Source: CAD feature listing. Evaluate the final solid. Frame: model axes, mm. A direction names the side the tool comes from. Round coordinates to 2 decimals unless told otherwise and drop trailing zeros. Order: outer loops, then holes, each group sorted by start corner. A loop starts at its lowest first (then second) coordinate and runs counter-clockwise, first axis right, second up. Notation, with made-up numbers: (27.5, 22) -> (62.5, 22) arc R16 ccw to (62.5, 27) -> close; hole circle Ø10 at (29.25, 61). An arc over 180 degrees is marked (long way). Write item = value, one per line. Start each with the question number.
(1) Ray query, line 1 (Z direction, x = 0, y = 1.8); line 2 (X direction, y = 2.8, z = 30); line 3 (X direction, y = 4.25, z = -30). Return the intervals inside material, ascending.
(2) Cut plane B-B on z = 0. Return the cut outline in (x, y), then the cut area to 3 significant figures.
(3) Draft query along X for faces 3 (the face through (-6.5, 6, -1)), 4 (the face through (0, 3, -40)), 5 (the face through (9.888, 6.147, -39.857)). Return one class per face: released by +X, released by -X, zero draft, split by the parting line, or undercut.
(4) Reachability of faces 1 (the face through (-9.888, 6.147, 39.857)), 2 (the face through (-3, 4, 1)) from +Z, -Z, +X, -X, +Y, -Y: full face, straight path, thin tool, end or side. Return the list, or none.
(5) Cut plane D-D on z = -22.5. Return the cut outline in (x, y).
(6) Cut plane A-A on x = 0. Give the number of separate pieces and of enclosed holes in the cut face, then the cut area to 3 significant figures.
(7) Contact query for flat-ended pins moving along their axis: pin 1 Ø4 at (x, z) = (1, 6) entering from +Y; pin 2 Ø2 at (y, z) = (5.5, -12) entering from -X; pin 3 Ø4.5 at (x, z) = (0, -30) entering from +Y. Output: stop coordinate, or through.
(8) Cut plane C-C on y = 2.5. Return the cut outline in (x, z), then the cut area to 3 significant figures.
from build123d import *

# Parameters (mm, degrees)
F0_W           = 12
F0_H           = 80
F0_R           = 2
F0_W_2         = 5
F0_W_3         = 0.5
F1_DEPTH       = 4
F2_DEPTH       = 8.5
F3_SIZE2       = 3
F3_SIZE        = 4.5
F4_SIZE2       = 3
F4_SIZE        = 4.5
F5_D           = 4
F5_CSINK_D     = 6
F5_CSINK_ANGLE = 90
F6_R           = 0.5


with BuildPart() as f1:
    # F0 (on Front) → F1 (new body)
    with BuildSketch(Plane.XZ):
        Rectangle(F0_W, F0_H)
        with Locations((0, -30)):
            Circle(F0_R, mode=Mode.SUBTRACT)
        Circle(F0_R, mode=Mode.SUBTRACT)
        with Locations((0, 30)):
            Circle(F0_R, mode=Mode.SUBTRACT)
        with Locations((-9, 0)):
            Rectangle(F0_W_2, F0_H)
        with Locations((-6.25, 0)):
            Rectangle(F0_W_3, F0_H)
        with Locations((6.25, 0)):
            Rectangle(F0_W_3, F0_H)
        with Locations((9, 0)):
            Rectangle(F0_W_2, F0_H)
    extrude(amount=-F1_DEPTH)

    # F0 (on Front) → F2 (join)
    with BuildSketch(Plane.XZ):
        with Locations((-9, 0)):
            Rectangle(F0_W_2, F0_H)
        with Locations((9, 0)):
            Rectangle(F0_W_2, F0_H)
    extrude(amount=-F2_DEPTH)

    # F3
    f3_edges = [f1.edges().sort_by_distance(p)[0] for p in [
        (-11.5, 8.5, 0),
    ]]
    f3_side = f1.faces().sort_by_distance((-11.5, 4.25, 0))[0]
    chamfer(f3_edges, length=F3_SIZE, length2=F3_SIZE2, reference=f3_side)

    # F4
    f4_edges = [f1.edges().sort_by_distance(p)[0] for p in [
        (11.5, 8.5, 0),
    ]]
    f4_side = f1.faces().sort_by_distance((11.5, 4.25, 0))[0]
    chamfer(f4_edges, length=F4_SIZE, length2=F4_SIZE2, reference=f4_side)

    # F5 (through all)
    with Locations(Plane.XZ):
        with Locations((0, 0), (0, -30), (0, 30)):
            CounterSinkHole(F5_D / 2, F5_CSINK_D / 2, counter_sink_angle=F5_CSINK_ANGLE)

    # F6
    f6_edges = [f1.edges().sort_by_distance(p)[0] for p in [
        (10, 6.25, -40),
        (11.5, 4, 0),
        (8.5, 8.5, 0),
        (10, 6.25, 40),
        (7.5, 8.5, -40),
        (6.5, 8.5, 0),
        (7.5, 8.5, 40),
        (-7.5, 8.5, -40),
        (-8.5, 8.5, 0),
        (-6.5, 8.5, 0),
        (-7.5, 8.5, 40),
        (-10, 6.25, 40),
        (-11.5, 4, 0),
        (-10, 6.25, -40),
        (-2, 4, -30),
        (-2, 4, 0),
        (0, 4, -40),
        (6.5, 6.25, -40),
        (-6.5, 6.25, -40),
        (-11.5, 2, -40),
        (11.5, 2, -40),
        (11.5, 2, 40),
        (6.5, 6.25, 40),
        (0, 4, 40),
        (-6.5, 6.25, 40),
        (-11.5, 2, 40),
        (-2, 4, 30),
    ]]
    fillet(f6_edges, radius=F6_R)


solid = f1.part
Evaluation:
q1.line_1 = -40 to -32, -28 to -2, 2 to 28, 32 to 40
q1.line_2 = -11.5 to -2, 2 to 11.5
q1.line_3 = -11.33 to -6.5, 6.5 to 11.33
q2.outline = (-11.5, 0) -> (-3, 0) -> (-2, 1) -> (-2, 3.5) arc R0.5 ccw to (-2.5, 4) -> (-6.5, 4) -> (-6.5, 8) arc R0.5 ccw to (-7, 8.5) -> (-8.23, 8.5) arc R0.5 ccw to (-8.65, 8.28) -> (-11.42, 4.13) arc R0.5 ccw to (-11.5, 3.85) -> close; (2, 1) -> (3, 0) -> (11.5, 0) -> (11.5, 3.85) arc R0.5 ccw to (11.42, 4.13) -> (8.65, 8.28) arc R0.5 ccw to (8.23, 8.5) -> (7, 8.5) arc R0.5 ccw to (6.5, 8) -> (6.5, 4) -> (2.5, 4) arc R0.5 ccw to (2, 3.5) -> close
q2.area = 106 mm^2
q3.face_3 = undercut
q3.face_4 = zero draft
q3.face_5 = released by +X
q4.face_1 = +Z, -X, +Y
q4.face_2 = +Z, -Z, +Y
q5.outline = (-11.5, 0) -> (11.5, 0) -> (11.5, 3.85) arc R0.5 ccw to (11.42, 4.13) -> (8.65, 8.28) arc R0.5 ccw to (8.23, 8.5) -> (7, 8.5) arc R0.5 ccw to (6.5, 8) -> (6.5, 4) -> (-6.5, 4) -> (-6.5, 8) arc R0.5 ccw to (-7, 8.5) -> (-8.23, 8.5) arc R0.5 ccw to (-8.65, 8.28) -> (-11.42, 4.13) arc R0.5 ccw to (-11.5, 3.85) -> close
q6.separate_pieces = 4
q6.enclosed_holes = 0
q6.area = 269 mm^2
q7.pin_1 = 4
q7.pin_2 = -11.17
q7.pin_3 = 3.93
q8.outline = (-11.5, -39.5) arc R0.5 ccw to (-11, -40) -> (11, -40) arc R0.5 ccw to (11.5, -39.5) -> (11.5, 39.5) arc R0.5 ccw to (11, 40) -> (-11, 40) arc R0.5 ccw to (-11.5, 39.5) -> close; hole circle Ø4 at (0, -30); hole circle Ø4 at (0, 0); hole circle Ø4 at (0, 30)
q8.area = 1,800 mm^2
